from build123d import *

# Parameters (mm, degrees)
PAD_DEPTH       = 40
SKETCH001_W     = 95
SKETCH001_H     = 40
PAD001_DEPTH    = 110
SKETCH002_R     = 20
SKETCH002_R_2   = 15
PAD002_DEPTH    = 8
SKETCH003_R     = 15
POCKET_DEPTH    = 40.001
FILLET_R        = 15
POCKET001_DEPTH = 40.001
POCKET002_DEPTH = 95.001
SKETCH006_R     = 5
POCKET003_DEPTH = 95.001


with BuildPart() as part:
    # Sketch → Pad (new body)
    with BuildSketch(Plane.XZ):
        with BuildLine():
            Line((47.5, 132.49995), (47.5, 0))
            Line((47.5, 0), (-47.5, 0))
            Line((-47.5, 0), (-47.5, 132.49995))
            ThreePointArc((47.5, 132.49995), (0, 180), (-47.5, 132.49995))
        make_face()
    extrude(amount=PAD_DEPTH)

    # Sketch001 → Pad001 (new body)
    with BuildSketch(Plane.XZ.offset(40)):
        with Locations((0, 20)):
            Rectangle(SKETCH001_W, SKETCH001_H)
    extrude(amount=PAD001_DEPTH)

    # Sketch002 → Pad002 (new body)
    with BuildSketch(Plane.XZ.offset(40)):
        with Locations((0, 132.5)):
            Circle(SKETCH002_R)
        with Locations((0, 132.5)):
            Circle(SKETCH002_R_2, mode=Mode.SUBTRACT)
    extrude(amount=PAD002_DEPTH)

    # Sketch003 → Pocket (cut, through all)
    with BuildSketch(Plane.XZ.offset(40)):
        with Locations((0, 132.5)):
            Circle(SKETCH003_R)
    extrude(amount=-POCKET_DEPTH, mode=Mode.SUBTRACT)

    # Fillet
    fillet_edges = [part.edges().sort_by_distance(p)[0] for p in [
        (0, -40, 40),
    ]]
    fillet(fillet_edges, radius=FILLET_R)

    # Sketch004 → Pocket001 (cut, through all)
    with BuildSketch(Plane(origin=(0, 0, 40), x_dir=(-1, 0, 0), z_dir=(0, 0, 1))):
        with BuildLine():
            ThreePointArc((-5, 129.364917), (-20, 110), (-5, 90.635083))
            Line((-5, 55), (-5, 90.635083))
            Line((5, 55), (-5, 55))
            Line((5, 90.635083), (5, 55))
            ThreePointArc((5, 90.635083), (20, 110), (5, 129.364917))
            Line((5, 129.364917), (5, 150))
            Line((5, 150), (-5, 150))
            Line((-5, 150), (-5, 129.364917))
        make_face()
    extrude(amount=-POCKET001_DEPTH, mode=Mode.SUBTRACT)

    # Sketch005 → Pocket002 (cut, through all)
    with BuildSketch(Plane(origin=(47.5, 0, 0), x_dir=(0, 0, 1), z_dir=(1, 0, 0))):
        Polygon((40, 150), (20, 150), (40, 75), align=None)
    extrude(amount=-POCKET002_DEPTH, mode=Mode.SUBTRACT)

    # Sketch006 → Pocket003 (cut, through all)
    with BuildSketch(Plane(origin=(47.5, 0, 0), x_dir=(0, 0, 1), z_dir=(1, 0, 0))):
        with Locations((10, 140)):
            Circle(SKETCH006_R)
    extrude(amount=-POCKET003_DEPTH, mode=Mode.SUBTRACT)


solid = part.part
Check sheet for the modelled part. Datum: model origin and axes. Units: mm. A direction names the side the tool comes from. Give positions to 0.01 mm unless a question says otherwise; leave off trailing zeros. Loops run counter-clockwise (first coordinate to the right, second up) from the corner with the lowest first, then second, coordinate; pieces in that order, holes last. Notation, with made-up numbers: M 12.5,4.25 L 25.5,4.25 A5 ccw 25.5,11.25 Z; hole C 24,-30.5 d9. An arc over 180 degrees is marked long. Answer as a JSON object with one key per item and string values. Group by question number.
Q1. Go/stop test with flat-tipped pins: P1, Ø2, axis at x = 34.5, z = 154.5, coming from the -Y side; P2, Ø22, axis at x = 36, y = -64, coming from the +Z side; P3, Ø5, axis at x = -1.5, z = 14, coming from the -Y side; P4, Ø24, axis at x = 0, z = 132.5, coming from the +Y side. Record where each tip stops, or that it passes through.
Q2. Cross-section at A-A on z = 10. Record the cut outline in (x, y).
Q3. Cross-section at C-C on y = -14. Record the cut outline in (x, z), then the cut area to 3 significant figures.
Q4. Access from +Z, -Z, +X, -X, +Y, -Y to the whole of each face (thin tool, end or side, straight path). Record for faces 1 (the flat face through (26, -65, 40)), 2 (the cylindrical face through (20, -110, 14)), 3 (the cylindrical face through (10.752, -43.944, 149.364)).
Q5. Cross-section at B-B on x = 0. Record the cut outline in (y, z).
Q6. Cross-section at D-D on x = 41. Record the cut outline in (y, z).
Q7. Material ranges on line 1 along Z through (x, y) = (0, -9.5); line 2 along X through (y, z) = (-44, 132); line 3 along Z through (x, y) = (0, -43), recorded low to high. Write a range as [from, to].
Q8. Release check for a two-part mould opening along X. For faces 4 (the flat face through (26, -150, 10)), 5 (the flat face through (-47.5, -41, 36)), 6 (the cylindrical face through (-20, -110, 14)), 7 (the flat face through (-5, -140, 16)) record: released by +X, released by -X, zero draft, split by the parting line, or undercut.
Evaluation:
{
 "1": {"P1": "stops at y = -40", "P2": "stops at z = 40.13", "P3": "stops at y = -55", "P4": "passes through"},
 "2": {"outline": "M -47.5,-150 L -5,-150 L -5,-145 L -47.5,-145 Z; M -47.5,-135 L -5,-135 L -5,-129.36 A20 cw -5,-90.64 L -5,-55 L 5,-55 L 5,-90.64 A20 cw 5,-129.36 L 5,-135 L 47.5,-135 L 47.5,0 L -47.5,0 Z; M 5,-150 L 47.5,-150 L 47.5,-145 L 5,-145 Z"},
 "3": {"outline": "M -47.5,0 L 47.5,0 L 47.5,132.5 A47.5 ccw -47.5,132.5 Z; hole C 0,132.5 d30", "area": "15,400 mm2"},
 "4": {"face 1": "+Z, +X, -X, -Y", "face 2": "+Z, -Z", "face 3": "-Y"},
 "5": {"outline": "M -55,0 L 0,0 L 0,117.5 L -48,117.5 L -48,112.5 L -40,112.5 L -40,55 A15 cw -55,40 Z; M -48,147.5 L 0,147.5 L 0,180 L -40,180 L -40,152.5 L -48,152.5 Z"},
 "6": {"outline": "M -150,0 L 0,0 L 0,156.48 L -40,156.48 L -40,55 A15 cw -55,40 L -75,40 L -150,20 Z; hole C -140,10 d10"},
 "7": {"line 1": "z = [0, 117.5], [147.5, 180]", "line 2": "x = [-19.99, -14.99], [14.99, 19.99]", "line 3": "z = [0, 46], [112.5, 117.5], [147.5, 152.5]"},
 "8": {"face 4": "zero draft", "face 5": "released by -X", "face 6": "undercut", "face 7": "undercut"}
}
